Could you check a few things on this model? Use its own coordinates, in mm. Give positions to 0.01 mm unless a question says otherwise; leave off trailing zeros. Loops run counter-clockwise (first coordinate to the right, second up) from the corner with the lowest first, then second, coordinate; pieces in that order, holes last. Notation, with made-up numbers: (62.25, 75.5) -> (119.25, 75.5) arc R25 cw to (119.25, 98.5) -> close; hole circle Ø6 at (6.5, 67). An arc over 180 degrees is marked (long way). Write each question's results on one line, items separated by ' | '. Start each with the question number.
Q1. If we section it at B-B, the plane x = -98: List the corners of the cut face in (y, z) for me, plus the area to 3 significant figures.
Q2. If we section it at A-A, the plane z = -24: List the corners of the cut face in (x, y) for me, plus the area to 3 significant figures.
Q3. If I drill on line 1 along X through (y, z) = (17, -41); line 2 along Z through (x, y) = (-101, 40); line 3 along X through (y, z) = (15, -29), over which ranges is the centre line in solid material (lowest first)?
from build123d import *

# Parameters (mm, degrees)
F1_DEPTH = 100.33


with BuildPart() as f1:
    # F0 (on Front) → F1 (new body)
    with BuildSketch(Plane.XZ):
        with BuildLine():
            Line((33.960865, -16.626953), (-86.174272, -16.626953))
            ThreePointArc((-86.174272, -16.626953), (-104.134784, -24.066441), (-111.574272, -42.026953))
            Line((-111.574272, -42.026953), (-111.574272, -92.826953))
            Line((-111.574272, -92.826953), (33.960865, -92.826953))
            Line((33.960865, -92.826953), (33.960865, -16.626953))
        make_face()
    extrude(amount=-F1_DEPTH)


solid = f1.part
Final values:
1) outline: (0, -92.83) -> (100.33, -92.83) -> (100.33, -19.55) -> (0, -19.55) -> close | area: 7,350 mm²
2) outline: (-104.07, 0) -> (33.96, 0) -> (33.96, 100.33) -> (-104.07, 100.33) -> close | area: 13,800 mm²
3) line 1: x = -111.55 to 33.96 | line 2: z = -92.83 to -21.4 | line 3: x = -107.98 to 33.96
